```python
from build123d import *

# Parameters (mm, degrees)
F1_DEPTH = 25.4
F2_W     = 12.7
F2_H     = 6.35
F3_DEPTH = 25.401
F4_W     = 12.7
F4_H     = 6.35
F5_DEPTH = 38.090076


with BuildPart() as f1:
    # F0 (on Front) → F1 (new body)
    with BuildSketch(Plane.XZ):
        Polygon((38.089076, 39.012315), (0, 38.1), (0, 0.912315), (38.089076, 0.912315), align=None)
    extrude(amount=F1_DEPTH)

    # F2 (on face) → F3 (cut, through all)
    with BuildSketch(Plane.XZ.offset(25.4)):
        with Locations((18.020797, 4.087315)):
            Rectangle(F2_W, F2_H)
    extrude(amount=-F3_DEPTH, mode=Mode.SUBTRACT)

    # F4 (on face) → F5 (cut, through all)
    with BuildSketch(Plane.YZ.offset(38.089076)):
        with Locations((-11.259039, 35.837315)):
            Rectangle(F4_W, F4_H)
    extrude(amount=-F5_DEPTH, mode=Mode.SUBTRACT)


solid = f1.part
```
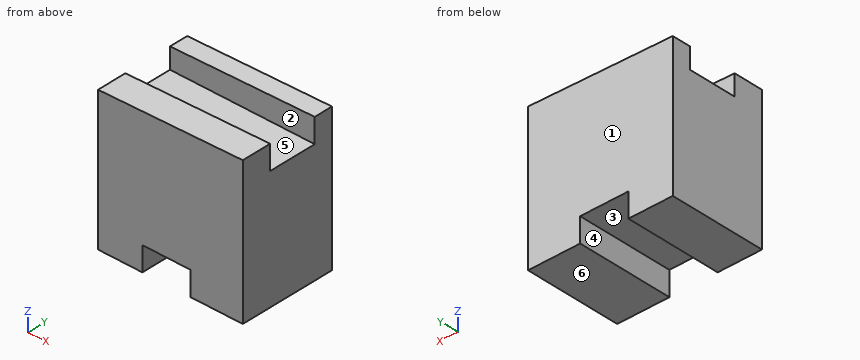
The model under review builds one solid part; all positions refer to its coordinate system, in mm. Face numbers are marked on the shaded views. A direction names the side the tool comes from. Round coordinates to 2 decimals unless told otherwise and drop trailing zeros. Write each loop counter-clockwise with the first axis right and the second up, starting at its lowest first coordinate (ties: lowest second). Pieces come first, ordered by that corner, then holes. Notation, with made-up numbers: M 34.5,15.25 L 63.5,15.25 A18 cw 63.5,45.25 Z; hole C -31,-27.5 d8. An arc over 180 degrees is marked long. Use CSV: the item, a comma, the result in double quotes. Start each with the question number.
(1) Tool access review of the marked faces 4, 5 and 6: name each direction out of +Z, -Z, +X, -X, +Y, -Y from which nothing blocks a thin tool from reaching the whole face with its end or side.
(2) For line 1 along Y through (x, z) = (20, 34); line 2 along X through (y, z) = (-4.5, 3); line 3 along Z through (x, y) = (16.5, -10), list the stretches that pass through material, from the lowest coordinate up.
(3) Clearance check with flat-ended pins moving along their axes: P1, Ø10, axis at x = 19, y = -16, coming from the -Z side; P2, Ø4, axis at x = 15.5, y = -12, coming from the +Z side; P3, Ø2, axis at x = 8.5, y = -5, coming from the +Z side. State where each tip first meets the part, or that it passes through.
(4) We need section B-B, the plane y = -14. State the section outline as (x, z) points.
(5) We need section A-A, the plane z = 37. State the section outline as (x, y) points.
(6) The part is to be moulded in two halves that separate along Y. For the marked faces 1, 2 and 3, say which applies: +Y half, -Y half, draft (parallel to the pull), parting line (faces both ways), or undercut.
(7) We need section C-C, the plane x = 28. State the section outline as (y, z) points.
Findings:
1,face 4,"-Z, +Y, -Y"
1,face 5,"+Z, +X, -X"
1,face 6,"-Z, +X, -X, +Y, -Y"
2,line 1,"-25.4 to -17.61, -4.91 to 0"
2,line 2,"0 to 11.67, 24.37 to 38.09"
2,line 3,"7.26 to 32.66"
3,P1,"z = 7.26"
3,P2,"z = 32.66"
3,P3,"z = 38.33"
4,outline,"M 0,0.91 L 11.67,0.91 L 11.67,7.26 L 24.37,7.26 L 24.37,0.91 L 38.09,0.91 L 38.09,32.66 L 0,32.66 Z"
5,outline,"M 0,-25.4 L 38.09,-25.4 L 38.09,-17.61 L 0,-17.61 Z; M 0,-4.91 L 38.09,-4.91 L 38.09,0 L 0,0 Z"
6,face 1,"+Y half"
6,face 2,"undercut"
6,face 3,"draft"
7,outline,"M -25.4,0.91 L 0,0.91 L 0,38.77 L -4.91,38.77 L -4.91,32.66 L -17.61,32.66 L -17.61,38.77 L -25.4,38.77 Z"
